```python
from build123d import *

# Parameters (mm, degrees)
CHANFREIN1_SIZE = 1
CHANFREIN2_SIZE = 0.5


with BuildPart() as part:
    # Esquisse1 → Révolution1 (revolve)
    with BuildSketch(Plane.XY):
        Polygon((0, 0), (-18, 0), (-18, 4), (-2, 4), (-2, 19), (0, 19), align=None)
    revolve(axis=Axis((0, 0, 0), (0, 1, 0)))

    # Chanfrein1
    chanfrein1_edges = [part.edges().sort_by_distance(p)[0] for p in [
        (2, 4, 0),
    ]]
    chamfer(chanfrein1_edges, length=CHANFREIN1_SIZE)

    # Chanfrein2
    chanfrein2_edges = [part.edges().sort_by_distance(p)[0] for p in [
        (2, 19, 0),
    ]]
    chamfer(chanfrein2_edges, length=CHANFREIN2_SIZE)


solid = part.part
```
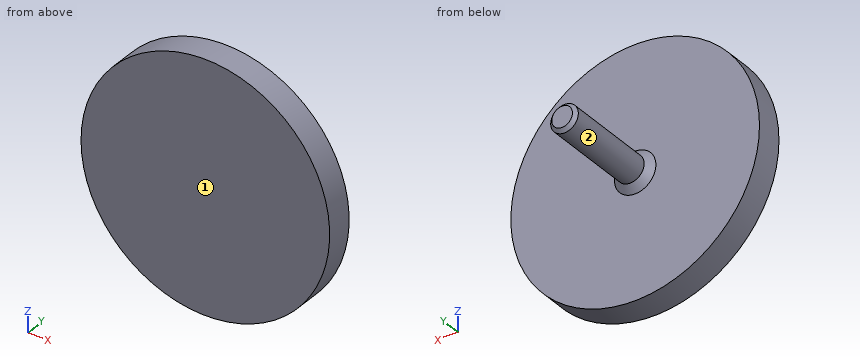
Here's how the part is built. I have some questions about the finished solid (model axes, mm). Face numbers are marked on the shaded views. A direction names the side the tool comes from. Coordinates: 2 decimals unless noted, no trailing zeros. Loops run counter-clockwise (first coordinate to the right, second up) from the corner with the lowest first, then second, coordinate; pieces in that order, holes last. Notation, with made-up numbers: M -35.75,-22.75 L -11.75,-22.75 A36 cw -11.75,11.25 Z; hole C 80.5,54.5 d5. An arc over 180 degrees is marked long. One line per item, written item: value.
1. On a 3-axis mill with a long thin cutter (end or side, diameter ignored), from which of +Z, -Z, +X, -X, +Y, -Y can I reach the whole of each face in a straight line? I mean the marked faces 1 and 2. Say none if no direction works.
Geometry says:
face 1: +Z, -Z, +X, -X, -Y
face 2: +Y
2. Imagine slicing it at C-C (y = 4.5). List the corners of the cut face in (x, z) for me.
Geometry says:
outline: C 0,0 d5
3. Please list where these lines run through material, in increasing order: probe 1 along Y at (x, z) = (-7, 5.5); probe 2 along Z at (x, y) = (0, 2); probe 3 along X at (y, z) = (16, 1.5).
Geometry says:
probe 1: y = 0 to 4
probe 2: z = -18 to 18
probe 3: x = -1.32 to 1.32
4. Imagine slicing it at A-A (x = 0). List the corners of the cut face in (y, z) for me.
Geometry says:
outline: M 0,-18 L 4,-18 L 4,-3 L 5,-2 L 18.5,-2 L 19,-1.5 L 19,1.5 L 18.5,2 L 5,2 L 4,3 L 4,18 L 0,18 Z
5. Will these pins go through, and if not, where does the flat tip stop? pin 1 Ø4 at (x, z) = (-3, 7) entering from +Y; pin 2 Ø5 at (y, z) = (5, -8) entering from +X.
Geometry says:
pin 1: stops at y = 4
pin 2: stops at x = 17.07
6. Imagine slicing it at B-B (z = 0). List the corners of the cut face in (x, y) for me.
Geometry says:
outline: M -18,0 L 18,0 L 18,4 L 3,4 L 2,5 L 2,18.5 L 1.5,19 L -1.5,19 L -2,18.5 L -2,5 L -3,4 L -18,4 Z
7. Imagine slicing it at D-D (y = 7). List the corners of the cut face in (x, z) for me.
Geometry says:
outline: C 0,0 d4
